Model file for the job. Use its own axes, mm. A direction names the side the tool comes from. Round coordinates to 2 decimals unless told otherwise and drop trailing zeros. Loops run counter-clockwise (first coordinate to the right, second up) from the corner with the lowest first, then second, coordinate; pieces in that order, holes last. Notation, with made-up numbers: M 43.25,-14 L 48.25,-14 A31 ccw 48.25,11 Z; hole C 15.5,-38 d1. An arc over 180 degrees is marked long. Answer in a Markdown table with one row per item.
from build123d import *

# Parameters (mm, degrees)
EXTRUDE_1_DEPTH     = 12
CUT_EXTRUDE_1_DEPTH = 9
SKETCH_3_R          = 2.25
CUT_EXTRUDE_2_DEPTH = 20


with BuildPart() as part:
    # Эскиз1 → Бобышка-Вытянуть1 (new body)
    with BuildSketch(Plane(origin=(0, 0, 0), x_dir=(0, 0, -1), z_dir=(1, 0, 0))):
        with BuildLine():
            Line((0, 2), (0, -4))
            Line((0, -4), (27, -4))
            Line((27, -4), (27, -2))
            Line((27, -2), (25, -2))
            ThreePointArc((25, -2), (23, 0), (25, 2))
            Line((25, 2), (29, 2))
            Line((29, 2), (29, 4))
            Line((29, 4), (23, 4))
            Line((23, 4), (0, 2))
        make_face()
    extrude(amount=EXTRUDE_1_DEPTH)

    # Эскиз2 → Вырез-Вытянуть1 (cut, through all)
    with BuildSketch(Plane(origin=(0, 4, 0), x_dir=(1, 0, 0), z_dir=(0, 1, 0))):
        Polygon((0, 0), (0, 20), (3, 0), align=None)
        Polygon((12, 20), (9, 0), (12, 0), align=None)
    extrude(amount=-CUT_EXTRUDE_1_DEPTH, mode=Mode.SUBTRACT)

    # Эскиз3 → Вырез-Вытянуть2 (cut)
    with BuildSketch(Plane.XY):
        with Locations((6, -1)):
            Circle(SKETCH_3_R)
    extrude(amount=-CUT_EXTRUDE_2_DEPTH, mode=Mode.SUBTRACT)


solid = part.part
1. Pin check, flat tips, straight feed: pin 1 (2 mm diameter, centred on x = 8, z = -8.5, fed in from +Y); pin 2 (3.5 mm diameter, centred on x = 6, y = -1, fed in from +Z); pin 3 (4 mm diameter, centred on x = 4, z = -6.5, fed in from +Y). Stop position of each tip, or through.
Verdict:
| item | result |
|---|---|
| pin 1 | stops at y = 2.83 |
| pin 2 | stops at z = -20 |
| pin 3 | stops at y = 2.74 |
2. Saw through at C-C (y = -1). Write the cut outline in (x, z), and give its area (3 significant figures).
Verdict:
| item | result |
|---|---|
| outline | M 0,-23.27 L 12,-23.27 L 12,-20 L 9,0 L 8.25,0 L 8.25,-20 L 3.75,-20 L 3.75,0 L 3,0 L 0,-20 Z |
| area | 129 mm² |
3. Saw through at D-D (z = -15.5). Write the cut outline in (x, y) (3 decimals).
Verdict:
| item | result |
|---|---|
| outline | M 0.675,-4 L 11.325,-4 L 11.325,3.348 L 0.675,3.348 Z; hole C 6,-1 d4.5 |
4. Tool access for faces 4 (the flat face through (6, -3, -27)), 5 (the flat face through (6, -1, -20)), 6 (the flat face through (6, 2, -27)): list every direction of +Z, -Z, +X, -X, +Y, -Y with a clear straight run to the whole face (end or side of a thin tool).
Verdict:
| item | result |
|---|---|
| face 4 | -Z, +X, -X, -Y |
| face 5 | +Z |
| face 6 | -Z, +X, -X |
5. Wall check: probe 1 along Y at (x, z) = (6, -11.5); probe 2 along Y at (x, z) = (1, -28); probe 3 along Y at (x, z) = (4.75, -15.5). Give the ranges that are in metal, low to high.
Verdict:
| item | result |
|---|---|
| probe 1 | y = -4 to -3.25, 1.25 to 3 |
| probe 2 | y = 2 to 4 |
| probe 3 | y = -4 to -2.87, 0.87 to 3.35 |
6. Saw through at A-A (x = 6). Write the cut outline in (y, z).
Verdict:
| item | result |
|---|---|
| outline | M -4,-27 L -2,-27 L -2,-25 A2 cw 2,-25 L 2,-29 L 4,-29 L 4,-23 L 2,0 L 1.25,0 L 1.25,-20 L -3.25,-20 L -3.25,0 L -4,0 Z |
7. Mould opens along Y. For faces 1 (the flat face through (5.916, 3.236, -14.217)), 2 (the cylindrical face through (8.146, -0.324, -9.86)), 3 (the flat face through (0, 0, -22)) say: +Y half, -Y half, draft (parallel to the pull), parting line (faces both ways), or undercut.
Verdict:
| item | result |
|---|---|
| face 1 | +Y half |
| face 2 | undercut |
| face 3 | draft |
8. Saw through at B-B (z = -19.5). Write the cut outline in (x, y) (3 decimals).
Verdict:
| item | result |
|---|---|
| outline | M 0.075,-4 L 11.925,-4 L 11.925,3.696 L 0.075,3.696 Z; hole C 6,-1 d4.5 |
